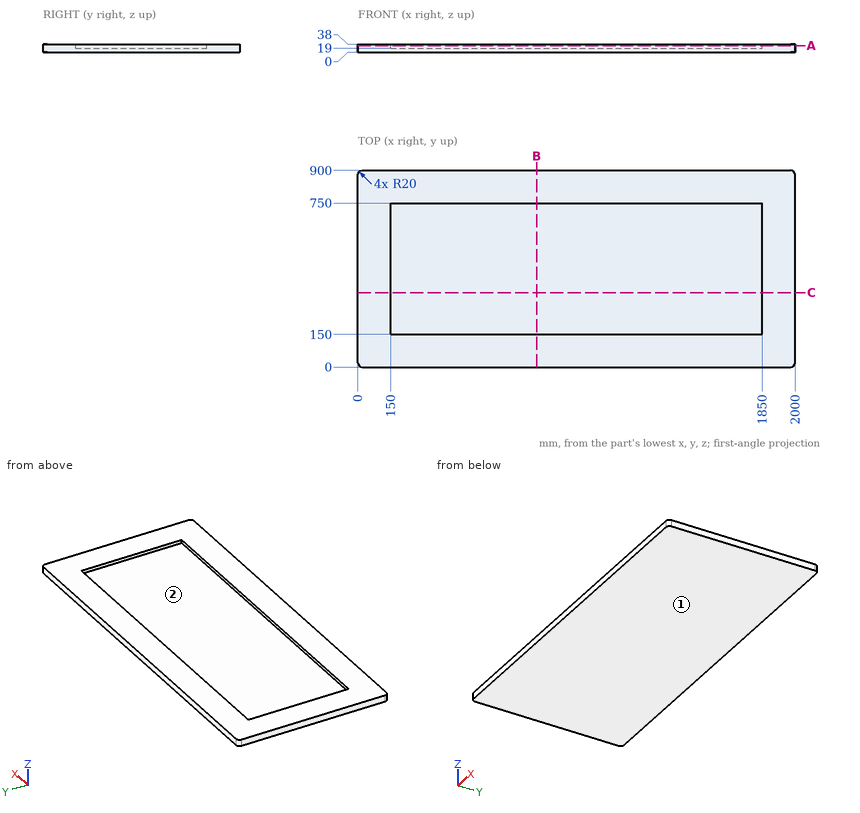
Here's the drawing with two shaded views (mm, measured from the low corner). I have some questions. A direction names the side the tool comes from. Coordinates: 2 decimals unless noted, no trailing zeros. Order: outer loops, then holes, each group sorted by start corner. A loop starts at its lowest first (then second) coordinate and runs counter-clockwise, first axis right, second up.
Item 1: If we section it at B-B on x = 818: List the corners of the cut face in (y, z) for me, plus the area to 3 significant figures.
Result sheet:
outline: (0, 0) - (900, 0) - (900, 38) - (750, 38) - (750, 19) - (150, 19) - (150, 38) - (0, 38) - close
area: 22,800 mm2
Item 2: For the marked faces 1 and 2, which set-ups out of +Z, -Z, +X, -X, +Y, -Y let a thin tool reach every point of the face, with its end or its side?
Result sheet:
face 1: -Z, +X, -X, +Y, -Y
face 2: +Z
Item 3: If we section it at A-A on z = 30: List the corners of the cut face in (x, y) for me.
Result sheet:
outline: (0, 20) arc R20 ccw to (20, 0) - (1980, 0) arc R20 ccw to (2000, 20) - (2000, 880) arc R20 ccw to (1980, 900) - (20, 900) arc R20 ccw to (0, 880) - close; hole (150, 150) - (1850, 150) - (1850, 750) - (150, 750) - close
Item 4: If we section it at C-C on y = 341: List the corners of the cut face in (x, z) for me, plus the area to 3 significant figures.
Result sheet:
outline: (0, 0) - (2000, 0) - (2000, 38) - (1850, 38) - (1850, 19) - (150, 19) - (150, 38) - (0, 38) - close
area: 43,700 mm2
Item 5: I need wall thicknesses on line 1 (X direction, y = 261, z = 31); line 2 (Y direction, x = 267, z = 34.5); line 3 (Z direction, x = 559, y = 577.5). Which ranges of each line are inside material? Lowest first, please.
Result sheet:
line 1: x = 0 to 150, 1850 to 2000
line 2: y = 0 to 150, 750 to 900
line 3: z = 0 to 19
